Source: CAD feature listing. Evaluate the final solid. Frame: model axes, mm. Face numbers are marked on the shaded views. Coordinates: 2 decimals unless noted, no trailing zeros. Loops run counter-clockwise (first coordinate to the right, second up) from the corner with the lowest first, then second, coordinate; pieces in that order, holes last. Notation, with made-up numbers: (-22.5, 66) -> (-13.5, 66) arc R22 ccw to (-13.5, 83) -> close; hole circle Ø5 at (89.5, 2.25). An arc over 180 degrees is marked (long way). Answer as a JSON object with one key per item and string values. Group by question number.
from build123d import *

# Parameters (mm, degrees)
SKETCH1_W           = 40
SKETCH1_H           = 10
BOSS_EXTRUDE1_DEPTH = 6
SKETCH2_R           = 2.25
CUT_EXTRUDE1_DEPTH  = 6
FILLET1_R           = 5
CHAMFER1_SIZE       = 0.6


with BuildPart() as part:
    # Sketch1 → Boss-Extrude1 (new body)
    with BuildSketch(Plane.XY):
        Rectangle(SKETCH1_W, SKETCH1_H)
    extrude(amount=BOSS_EXTRUDE1_DEPTH)

    # Sketch2 → Cut-Extrude1 (cut)
    with BuildSketch(Plane.XY.offset(6)):
        with Locations((-12, 0)):
            Circle(SKETCH2_R)
        with Locations(Location((12, 0, 0), (0, 0, 180))):
            Circle(SKETCH2_R)
    extrude(amount=-CUT_EXTRUDE1_DEPTH, mode=Mode.SUBTRACT)

    # Fillet1
    fillet1_edges = [part.edges().sort_by_distance(p)[0] for p in [
        (20, -5, 3),
        (20, 5, 3),
        (-20, -5, 3),
        (-20, 5, 3),
    ]]
    fillet(fillet1_edges, radius=FILLET1_R - 0.0001)  # a hair under: the kernel refuses the full size

    # Chamfer1
    chamfer1_edges = [part.edges().sort_by_distance(p)[0] for p in [
        (0, -5, 0),
        (0, 5, 0),
        (-18.535563195, 3.535563195, 0),
        (-18.535563195, -3.535563195, 0),
        (18.535563195, 3.535563195, 0),
        (18.535563195, -3.535563195, 0),
        (0, -5, 6),
        (0, 5, 6),
        (-18.535563195, 3.535563195, 6),
        (-18.535563195, -3.535563195, 6),
        (18.535563195, 3.535563195, 6),
        (18.535563195, -3.535563195, 6),
    ]]
    chamfer(chamfer1_edges, length=CHAMFER1_SIZE)


solid = part.part
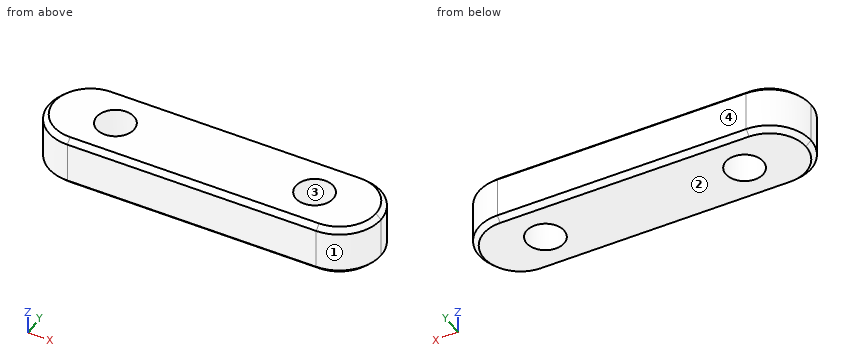
1. Section query B-B on z = 2.75. State how many separate pieces and enclosed holes the cut face has, then the cut area to 3 significant figures.
2. Ray query, L1, parallel to Y at x = -12, z = 3.2; L2, parallel to X at y = -1.25, z = 4.75; L3, parallel to X at y = -1, z = 3. Return the intervals inside material, ascending.
3. Pin query (flat end, axial travel): pin 1 Ø2.5 at (x, y) = (-12, 0) entering from -Z. Return the tip coordinate at first contact, or that it passes through.
4. Mould query, pull axis Y, two halves, no side actions, for the marked faces 1, 2, 3 and 4. Classes: pulls with the +Y half, pulls with the -Y half, needs draft (parallel to the pull), parting line crosses it, or undercut.
5. Section query A-A on x = -12. Return loops of the section in (y, z), then the cut area to 3 significant figures.
Solved:
{
 "1": {"separate pieces": "1", "enclosed holes": "2", "area": "347 mm^2"},
 "2": {"L1": "-5 to -2.25, 2.25 to 5", "L2": "-19.84 to -13.87, -10.13 to 10.13, 13.87 to 19.84", "L3": "-19.9 to -14.02, -9.98 to 9.98, 14.02 to 19.9"},
 "3": {"pin 1": "through"},
 "4": {"face 1": "pulls with the -Y half", "face 2": "needs draft", "face 3": "undercut", "face 4": "pulls with the +Y half"},
 "5": {"outline": "(-5, 0.6) -> (-4.4, 0) -> (-2.25, 0) -> (-2.25, 6) -> (-4.4, 6) -> (-5, 5.4) -> close; (2.25, 0) -> (4.4, 0) -> (5, 0.6) -> (5, 5.4) -> (4.4, 6) -> (2.25, 6) -> close", "area": "32.3 mm^2"}
}
